Check sheet for the modelled part. Datum: model origin and axes. Units: mm. Face numbers are marked on the shaded views. A direction names the side the tool comes from. Round coordinates to 2 decimals unless told otherwise and drop trailing zeros. Order: outer loops, then holes, each group sorted by start corner. A loop starts at its lowest first (then second) coordinate and runs counter-clockwise, first axis right, second up. Notation, with made-up numbers: M 88.25,79 L 104.25,79 A26 ccw 104.25,96 Z; hole C 75.25,9.5 d8. An arc over 180 degrees is marked long. One line per item, written item: value. Start each with the question number.
(1) Cross-section at A-A, the plane z = 0. Enter the section's corners in (x, y).
(2) Release check for a two-part mould opening along Z. For the marked faces 1 and 2 record: released by +Z, released by -Z, zero draft, split by the parting line, or undercut.
(3) Thickness scan on L1, parallel to Z at x = 17.5, y = 35.5; L2, parallel to X at y = 43, z = 33; L3, parallel to X at y = 22.5, z = -47.5. Record the ranges inside material, lowest first.
(4) Cross-section at C-C, the plane x = 11.25. Enter the section's corners in (y, z), and give its area (3 significant figures).
(5) Cross-section at D-D, the plane y = 15.5. Enter the section's corners in (x, z).
(6) Depth check by flat-ended pin: pin 1 Ø10.5 at (y, z) = (51.27, -51.27) entering from +X; pin 2 Ø8 at (x, z) = (17, -15.5) entering from -Y; pin 3 Ø3 at (x, y) = (20, 27.5) entering from +Z; pin 4 Ø19 at (y, z) = (0, 0) entering from -X. Enter the tip coordinate at first touch or a pass-through.
(7) Access from +Z, -Z, +X, -X, +Y, -Y to the whole of each face (thin tool, end or side, straight path). Record for the marked faces 3, 4 and 5.
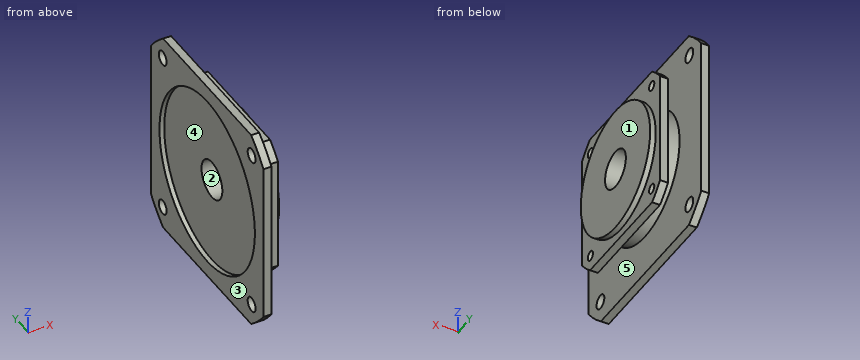
from build123d import *

# Parameters (mm, degrees)
SKETCH_1_R          = 4.5
EXTRUDE_1_DEPTH     = 5
SKETCH_2_R          = 55
CUT_EXTRUDE_1_DEPTH = 3
SKETCH_3_R          = 40
EXTRUDE_2_DEPTH     = 10
SKETCH_4_R          = 3
EXTRUDE_3_DEPTH     = 5
SKETCH_5_R          = 40
EXTRUDE_4_DEPTH     = 3.5
SKETCH_6_R          = 12
CUT_EXTRUDE_2_DEPTH = 95.880187605


with BuildPart() as part:
    # 草图1 → 凸台-拉伸1 (new body)
    with BuildSketch(Plane(origin=(0, 0, 0), x_dir=(0, 0, -1), z_dir=(1, 0, 0))):
        with BuildLine():
            Line((50.806003582, -65), (-50.806003582, -65))
            ThreePointArc((-50.806003582, -65), (-58.336309448, -58.336309448), (-65, -50.806003582))
            Line((-65, -50.806003582), (-65, 50.806003582))
            ThreePointArc((-65, 50.806003582), (-58.336309448, 58.336309448), (-50.806003582, 65))
            Line((-50.806003582, 65), (50.806003582, 65))
            ThreePointArc((50.806003582, 65), (58.336309448, 58.336309448), (65, 50.806003582))
            Line((65, 50.806003582), (65, -50.806003582))
            ThreePointArc((65, -50.806003582), (58.336309448, -58.336309448), (50.806003582, -65))
        make_face()
        with Locations((-51.265241636, 51.265241636)):
            Circle(SKETCH_1_R, mode=Mode.SUBTRACT)
        with Locations(Location((51.265241636, -51.265241636, 0), (0, 0, 180))):
            Circle(SKETCH_1_R, mode=Mode.SUBTRACT)
        with Locations((51.265241636, 51.265241636)):
            Circle(SKETCH_1_R, mode=Mode.SUBTRACT)
        with Locations(Location((-51.265241636, -51.265241636, 0), (0, 0, 180))):
            Circle(SKETCH_1_R, mode=Mode.SUBTRACT)
    extrude(amount=EXTRUDE_1_DEPTH)

    # 草图2 → 切除-拉伸1 (cut)
    with BuildSketch(Plane.ZY):
        Circle(SKETCH_2_R)
    extrude(amount=-CUT_EXTRUDE_1_DEPTH, mode=Mode.SUBTRACT)

    # 草图3 → 凸台-拉伸2 (add)
    with BuildSketch(Plane(origin=(5, 0, 0), x_dir=(0, 0, -1), z_dir=(1, 0, 0))):
        Circle(SKETCH_3_R)
    extrude(amount=EXTRUDE_2_DEPTH)

    # 草图4 → 凸台-拉伸3 (add)
    with BuildSketch(Plane(origin=(15, 0, 0), x_dir=(0, 0, -1), z_dir=(1, 0, 0))):
        with BuildLine():
            Line((35.794552658, -45), (-35.794552658, -45))
            ThreePointArc((-35.794552658, -45), (-40.658639918, -40.658639918), (-45, -35.794552658))
            Line((-45, -35.794552658), (-45, 35.794552658))
            ThreePointArc((-45, 35.794552658), (-40.658639918, 40.658639918), (-35.794552658, 45))
            Line((-35.794552658, 45), (35.794552658, 45))
            ThreePointArc((35.794552658, 45), (40.658639918, 40.658639918), (45, 35.794552658))
            Line((45, 35.794552658), (45, -35.794552658))
            ThreePointArc((45, -35.794552658), (40.658639918, -40.658639918), (35.794552658, -45))
        make_face()
        with Locations((-35.355339059, 35.355339059)):
            Circle(SKETCH_4_R, mode=Mode.SUBTRACT)
        with Locations(Location((35.355339059, -35.355339059, 0), (0, 0, 180))):
            Circle(SKETCH_4_R, mode=Mode.SUBTRACT)
        with Locations((35.355339059, 35.355339059)):
            Circle(SKETCH_4_R, mode=Mode.SUBTRACT)
        with Locations(Location((-35.355339059, -35.355339059, 0), (0, 0, 180))):
            Circle(SKETCH_4_R, mode=Mode.SUBTRACT)
    extrude(amount=EXTRUDE_3_DEPTH)

    # 草图5 → 凸台-拉伸4 (add)
    with BuildSketch(Plane(origin=(20, 0, 0), x_dir=(0, 0, -1), z_dir=(1, 0, 0))):
        Circle(SKETCH_5_R)
    extrude(amount=EXTRUDE_4_DEPTH)

    # 草图6 → 切除-拉伸2 (cut, through all)
    with BuildSketch(Plane(origin=(23.5, 0, 0), x_dir=(0, 0, -1), z_dir=(1, 0, 0))):
        Circle(SKETCH_6_R)
    extrude(amount=-CUT_EXTRUDE_2_DEPTH, mode=Mode.SUBTRACT)


solid = part.part
Values found:
1. outline: M 0,-65 L 5,-65 L 5,-40 L 15,-40 L 15,-45 L 20,-45 L 20,-40 L 23.5,-40 L 23.5,-12 L 3,-12 L 3,-55 L 0,-55 Z; M 0,55 L 3,55 L 3,12 L 23.5,12 L 23.5,40 L 20,40 L 20,45 L 15,45 L 15,40 L 5,40 L 5,65 L 0,65 Z
2. face 1: zero draft
2. face 2: undercut
3. L1: -45 to -38.35, -32.36 to 32.36, 38.35 to 45
3. L2: 3 to 5, 15 to 20
3. L3: 3 to 5
4. outline: C 0,0 d80; hole C 0,0 d24
4. area: 4,570 mm^2
5. outline: M 0,-65 L 5,-65 L 5,-36.87 L 15,-36.87 L 15,-45 L 20,-45 L 20,-36.87 L 23.5,-36.87 L 23.5,36.87 L 20,36.87 L 20,45 L 15,45 L 15,36.87 L 5,36.87 L 5,65 L 0,65 L 0,52.77 L 3,52.77 L 3,-52.77 L 0,-52.77 Z
6. pin 1: x = 5
6. pin 2: y = -45
6. pin 3: z = 45
6. pin 4: through
7. face 3: +Z, -Z, -X, +Y, -Y
7. face 4: -X
7. face 5: none
